Model file for the job. Use its own axes, mm. A direction names the side the tool comes from. Round coordinates to 2 decimals unless told otherwise and drop trailing zeros. Write each loop counter-clockwise with the first axis right and the second up, starting at its lowest first coordinate (ties: lowest second). Pieces come first, ordered by that corner, then holes.
```python
from build123d import *

# Parameters (mm, degrees)
BOSS_EXTRUDE1_DEPTH      = 19.05
BOSS_EXTRUDE2_DEPTH      = 3.81
BOSS_EXTRUDE2_DEPTH_BACK = 3.81
BOSS_EXTRUDE2_START      = -9.525
SKETCH3_W                = 19.725995145
SKETCH3_H                = 15.0557617
SKETCH3_W_2              = 20.448664957
SKETCH3_H_2              = 15.24
BOSS_EXTRUDE3_DEPTH      = 2.54
SKETCH4_R                = 1.7526
CUT_EXTRUDE1_DEPTH       = 9.398


with BuildPart() as part:
    # Sketch1 → Boss-Extrude1 (new body)
    with BuildSketch(Plane.XY):
        with BuildLine():
            ThreePointArc((19.225490484, 2.284288075), (2.719598367, -0.626146046), (-13.78629375, 2.284288075))
            Line((-13.78629375, 2.284288075), (-14.655024914, -0.102531182))
            ThreePointArc((-14.655024914, -0.102531182), (2.719598367, -3.166146046), (20.094221648, -0.102531182))
            Line((20.094221648, -0.102531182), (19.225490484, 2.284288075))
        make_face()
    extrude(amount=BOSS_EXTRUDE1_DEPTH)

    # Sketch2 → Boss-Extrude2 (add, two sides: drawn at the far end of the back side and taken through both)
    with BuildSketch(Plane.XY.offset(19.05).offset(BOSS_EXTRUDE2_START - BOSS_EXTRUDE2_DEPTH_BACK)):
        with BuildLine():
            Line((51.959734492, -54.302617815), (20.094221648, -0.102531182))
            ThreePointArc((20.094221648, -0.102531182), (14.827776239, -1.702056179), (9.419193894, -2.722430855))
            Line((9.419193894, -2.722430855), (39.19902872, -54.302617815))
            Line((39.19902872, -54.302617815), (51.959734492, -54.302617815))
        make_face()
        with BuildLine():
            ThreePointArc((-3.979997159, -2.722430855), (-9.388579504, -1.702056179), (-14.655024914, -0.102531182))
            Line((-14.655024914, -0.102531182), (-45.947459522, -54.302617815))
            Line((-45.947459522, -54.302617815), (-33.759831986, -54.302617815))
            Line((-33.759831986, -54.302617815), (-3.979997159, -2.722430855))
        make_face()
    extrude(amount=BOSS_EXTRUDE2_DEPTH + BOSS_EXTRUDE2_DEPTH_BACK)

    # Sketch3 → Boss-Extrude3 (add)
    with BuildSketch(Plane.XZ.offset(54.302617815)):
        with Locations((-39.812829559, 9.514418368)):
            Rectangle(SKETCH3_W, SKETCH3_H)
        with Locations((45.545402014, 9.525)):
            Rectangle(SKETCH3_W_2, SKETCH3_H_2)
    extrude(amount=-BOSS_EXTRUDE3_DEPTH)

    # Sketch4 → Cut-Extrude1 (cut)
    with BuildSketch(Plane(origin=(0, 0, 0), x_dir=(1, 0, 0), z_dir=(0, 1, 0))):
        with Locations(Location((2.719598367, -3.236263, 0), (0, 0, 270))):
            Circle(SKETCH4_R)
        with Locations(Location((2.719598367, -15.875, 0), (0, 0, 270))):
            Circle(SKETCH4_R)
    extrude(amount=-CUT_EXTRUDE1_DEPTH, mode=Mode.SUBTRACT)


solid = part.part
```
1) Cut at C-C on z = 9. List the corners of the cut face in (x, y).
2) Cut at B-B on z = 15.25. List the corners of the cut face in (x, y).
3) Which spindle directions (+Z, -Z, +X, -X, +Y, -Y) get a long thin tool onto all of the face, cutting with end or side? Do faces 1 (the face through (-29.95, -53, 9)), 2 (the face through (2.471, -3.166, 9.392)), 3 (the face through (-40, -53, 17.042)). Say none if no direction does.
4) Cut at A-A on y = -32.5. List the corners of the cut face in (x, z) (3 decimals).
5) Flat gauge pins, fed straight in: pin 1 Ø6 at (y, z) = (-7, 8) entering from -X; pin 2 Ø3 at (x, y) = (40.5, -52.5) entering from +Z (3 decimals); pin 3 Ø3 at (x, y) = (-43.5, -52.5) entering from +Z. Where does each tip first touch, or does it go through?
6) Pull direction X, two halves, no side cores. Call faces 4 (the face through (45, -53, 17.145)), 5 (the face through (55.77, -53, 9)), 6 (the face through (-18.335, -27.586, 9.472)): released by +X, released by -X, zero draft, split by the parting line, or undercut.
7) Wall check: probe 1 along X at (y, z) = (-7, 9.5); probe 2 along Y at (x, z) = (39.5, 4.25); probe 3 along Z at (x, y) = (25, -13.5) (3 decimals). Give the ranges that are in metal, low to high.
8) Cut at D-D on x = 40. List the corners of the cut face in (y, z) (3 decimals), and give its area (3 significant figures).
Result sheet:
1. outline: (-49.68, -54.3) - (-29.95, -54.3) - (-29.95, -51.76) - (-32.29, -51.76) - (-3.98, -2.72) arc R50.8 ccw to (9.42, -2.72) - (37.73, -51.76) - (35.32, -51.76) - (35.32, -54.3) - (55.77, -54.3) - (55.77, -51.76) - (50.47, -51.76) - (20.09, -0.1) - (19.23, 2.28) arc R48.26 cw to (-13.79, 2.28) - (-14.66, -0.1) - (-44.48, -51.76) - (-49.68, -51.76) - close
2. outline: (-49.68, -54.3) - (-29.95, -54.3) - (-29.95, -51.76) - (-49.68, -51.76) - close; (-14.66, -0.1) arc R50.8 ccw to (1.08, -3.14) - (1.08, -0.6) arc R48.26 cw to (-13.79, 2.28) - close; (4.36, -3.14) arc R50.8 ccw to (20.09, -0.1) - (19.23, 2.28) arc R48.26 cw to (4.36, -0.6) - close; (35.32, -54.3) - (55.77, -54.3) - (55.77, -51.76) - (35.32, -51.76) - close
3. face 1: +Z, -Z, -Y
3. face 2: -Y
3. face 3: +Z, -X, +Y, -Y
4. outline: (-33.36, 5.715) - (-21.172, 5.715) - (-21.172, 13.335) - (-33.36, 13.335) - close; (26.611, 5.715) - (39.141, 5.715) - (39.141, 13.335) - (26.611, 13.335) - close
5. pin 1: stops at x = -20.37
5. pin 2: stops at z = 17.145
5. pin 3: stops at z = 17.04
6. face 4: zero draft
6. face 5: released by +X
6. face 6: undercut
7. probe 1: x = -18.64 to -6.45, 11.89 to 24.15
7. probe 2: y = -54.3 to -51.76
7. probe 3: z = 5.715 to 13.335
8. outline: (-54.303, 1.905) - (-51.763, 1.905) - (-51.763, 5.715) - (-33.96, 5.715) - (-33.96, 13.335) - (-51.763, 13.335) - (-51.763, 17.145) - (-54.303, 17.145) - close
8. area: 174 mm2
